CAD build for the part. Positions are in the model's coordinates, mm. A direction names the side the tool comes from. Coordinates: 2 decimals unless noted, no trailing zeros. Loops run counter-clockwise (first coordinate to the right, second up) from the corner with the lowest first, then second, coordinate; pieces in that order, holes last.
1) Which spindle directions (+Z, -Z, +X, -X, +Y, -Y) get a long thin tool onto all of the face, cutting with end or side? Do faces 1 (the flat face through (0, 0, 0)), 2 (the flat face through (-8.176, 3.933, -2.218)), 3 (the flat face through (0, 0, -4.5)). Say none if no direction does.
2) Pin check, flat tip, straight feed: pin 1 Ø12 at (x, y) = (-3.5, -5) entering from +Z. Stop position of the tip, or through.
3) Two-plate mould, pull along X, no slides. Class faces 4 (the flat face through (3.933, 8.176, -2.218)), 5 (the flat face through (-3.933, -8.176, -2.218)), 6 (the flat face through (-18, 0, -2)), 7 (the flat face through (-15, -17, 4)): +X half, -X half, draft (parallel to the pull), parting line (faces both ways), or undercut.
4) Saw through at B-B, the plane y = 11. Write the cut outline in (x, z).
5) Saw through at A-A, the plane z = -2. Give the number of separate pieces and of enclosed holes in the cut face, and give its area (3 significant figures).
6) Saw through at D-D, the plane y = -0.5. Write the cut outline in (x, z), and give its area (3 significant figures).
7) Wall check: line 1 along X through (y, z) = (-15, 2.4); line 2 along Y through (x, z) = (-15, -2.55). Give the ranges that are in metal, low to high.
8) Saw through at C-C, the plane x = -3. Write the cut outline in (y, z).
```python
from build123d import *
from build123d import SkipClean  # not in build123d's __all__

# Parameters (mm, degrees)
F1_W     = 36
F1_H     = 36
F2_DEPTH = 4.5
F3_DEPTH = 4


with BuildPart() as f2:
    # F1 (on Top) → F2 (new body)
    with BuildSketch(Plane.XY):
        Rectangle(F1_W, F1_H)
        with BuildLine():
            ThreePointArc((-15, 12.5), (-16.767766953, 16.767766953), (-12.5, 15))
            Line((-12.5, 15), (12.5, 15))
            ThreePointArc((12.5, 15), (15, 17.5), (17.5, 15))
            ThreePointArc((17.5, 15), (16.767766953, 13.232233047), (15, 12.5))
            Line((15, 12.5), (15, -12.5))
            ThreePointArc((15, -12.5), (16.767766953, -13.232233047), (17.5, -15))
            ThreePointArc((17.5, -15), (15, -17.5), (12.5, -15))
            Line((12.5, -15), (-12.5, -15))
            ThreePointArc((-12.5, -15), (-16.767766953, -16.767766953), (-15, -12.5))
            Line((-15, -12.5), (-15, 12.5))
        make_face(mode=Mode.SUBTRACT)
        with BuildLine():
            ThreePointArc((-13.232233047, 13.232233047), (-14.0432914191, 12.6903011687), (-15, 12.5))
            Line((-15, 12.5), (-15, -12.5))
            ThreePointArc((-15, -12.5), (-14.0432914191, -12.6903011687), (-13.232233047, -13.232233047))
            Line((-13.232233047, -13.232233047), (-12, -12))
            Line((-12, -12), (-12, -7.7573593129))
            Line((-12, -7.7573593129), (-12, 7.7573593129))
            Line((-12, 7.7573593129), (-12, 12))
            Line((-12, 12), (-13.232233047, 13.232233047))
        make_face()
        with BuildLine():
            Line((12.5, 15), (-12.5, 15))
            ThreePointArc((-12.5, 15), (-12.6903011687, 14.0432914191), (-13.232233047, 13.232233047))
            Line((-13.232233047, 13.232233047), (-12, 12))
            Line((-12, 12), (-7.7573593129, 12))
            Line((-7.7573593129, 12), (7.7573593129, 12))
            Line((7.7573593129, 12), (12, 12))
            Line((12, 12), (13.232233047, 13.232233047))
            ThreePointArc((13.232233047, 13.232233047), (12.6903011687, 14.0432914191), (12.5, 15))
        make_face()
        with BuildLine():
            Line((-12, -12), (-13.232233047, -13.232233047))
            ThreePointArc((-13.232233047, -13.232233047), (-12.6903011687, -14.0432914191), (-12.5, -15))
            Line((-12.5, -15), (12.5, -15))
            ThreePointArc((12.5, -15), (12.6903011687, -14.0432914191), (13.232233047, -13.232233047))
            Line((13.232233047, -13.232233047), (12, -12))
            Line((12, -12), (7.7573593129, -12))
            Line((7.7573593129, -12), (-7.7573593129, -12))
            Line((-7.7573593129, -12), (-12, -12))
        make_face()
        with BuildLine():
            ThreePointArc((15, 12.5), (14.0432914191, 12.6903011687), (13.232233047, 13.232233047))
            Line((13.232233047, 13.232233047), (12, 12))
            Line((12, 12), (12, 7.7573593129))
            Line((12, 7.7573593129), (12, -7.7573593129))
            Line((12, -7.7573593129), (12, -12))
            Line((12, -12), (13.232233047, -13.232233047))
            ThreePointArc((13.232233047, -13.232233047), (14.0432914191, -12.6903011687), (15, -12.5))
            Line((15, -12.5), (15, 12.5))
        make_face()
        Polygon((0, 0), (-12, 12), (-12, 7.7573593129), (-4.2426406871, 0), (-2.1213203436, -2.1213203436), align=None)
        Polygon((-7.7573593129, 12), (-12, 12), (0, 0), (2.1213203436, 2.1213203436), (0, 4.2426406871), align=None)
        Polygon((2.1213203436, 2.1213203436), (0, 0), (12, -12), (12, -7.7573593129), (4.2426406871, 0), align=None)
        Polygon((12, -12), (0, 0), (-2.1213203436, -2.1213203436), (0, -4.2426406871), (7.7573593129, -12), align=None)
        Polygon((-2.1213203436, -2.1213203436), (-12, -12), (-7.7573593129, -12), (0, -4.2426406871), align=None)
        Polygon((-12, -7.7573593129), (-12, -12), (-2.1213203436, -2.1213203436), (-4.2426406871, 0), align=None)
        Polygon((2.1213203436, 2.1213203436), (12, 12), (7.7573593129, 12), (0, 4.2426406871), align=None)
        Polygon((12, 7.7573593129), (12, 12), (2.1213203436, 2.1213203436), (4.2426406871, 0), align=None)
        with BuildLine():
            Line((-13.5, 15), (-12.5, 15))
            ThreePointArc((-12.5, 15), (-16.767766953, 16.767766953), (-15, 12.5))
            Line((-15, 12.5), (-15, 13.5))
            ThreePointArc((-15, 13.5), (-16.0606601718, 16.0606601718), (-13.5, 15))
        make_face()
        with BuildLine():
            ThreePointArc((17.5, 15), (15, 17.5), (12.5, 15))
            Line((12.5, 15), (13.5, 15))
            ThreePointArc((13.5, 15), (15, 16.5), (16.5, 15))
            ThreePointArc((16.5, 15), (16.0606601718, 13.9393398282), (15, 13.5))
            Line((15, 13.5), (15, 12.5))
            ThreePointArc((15, 12.5), (16.767766953, 13.232233047), (17.5, 15))
        make_face()
        with BuildLine():
            ThreePointArc((17.5, -15), (16.767766953, -13.232233047), (15, -12.5))
            Line((15, -12.5), (15, -13.5))
            ThreePointArc((15, -13.5), (16.0606601718, -13.9393398282), (16.5, -15))
            ThreePointArc((16.5, -15), (15, -16.5), (13.5, -15))
            Line((13.5, -15), (12.5, -15))
            ThreePointArc((12.5, -15), (15, -17.5), (17.5, -15))
        make_face()
        with BuildLine():
            Line((-15, -13.5), (-15, -12.5))
            ThreePointArc((-15, -12.5), (-16.767766953, -16.767766953), (-12.5, -15))
            Line((-12.5, -15), (-13.5, -15))
            ThreePointArc((-13.5, -15), (-16.0606601718, -16.0606601718), (-15, -13.5))
        make_face()
        with BuildLine():
            Line((-15, 13.5), (-15, 12.5))
            ThreePointArc((-15, 12.5), (-14.0432914191, 12.6903011687), (-13.232233047, 13.232233047))
            Line((-13.232233047, 13.232233047), (-13.9393398282, 13.9393398282))
            ThreePointArc((-13.9393398282, 13.9393398282), (-14.4259748515, 13.6141807012), (-15, 13.5))
        make_face()
        with BuildLine():
            ThreePointArc((-13.232233047, 13.232233047), (-12.6903011687, 14.0432914191), (-12.5, 15))
            Line((-12.5, 15), (-13.5, 15))
            ThreePointArc((-13.5, 15), (-13.6141807012, 14.4259748515), (-13.9393398282, 13.9393398282))
            Line((-13.9393398282, 13.9393398282), (-13.232233047, 13.232233047))
        make_face()
        with BuildLine():
            Line((13.9393398282, 13.9393398282), (13.232233047, 13.232233047))
            ThreePointArc((13.232233047, 13.232233047), (14.0432914191, 12.6903011687), (15, 12.5))
            Line((15, 12.5), (15, 13.5))
            ThreePointArc((15, 13.5), (14.4259748515, 13.6141807012), (13.9393398282, 13.9393398282))
        make_face()
        with BuildLine():
            Line((13.5, 15), (12.5, 15))
            ThreePointArc((12.5, 15), (12.6903011687, 14.0432914191), (13.232233047, 13.232233047))
            Line((13.232233047, 13.232233047), (13.9393398282, 13.9393398282))
            ThreePointArc((13.9393398282, 13.9393398282), (13.6141807012, 14.4259748515), (13.5, 15))
        make_face()
        with BuildLine():
            ThreePointArc((13.232233047, -13.232233047), (12.6903011687, -14.0432914191), (12.5, -15))
            Line((12.5, -15), (13.5, -15))
            ThreePointArc((13.5, -15), (13.6141807012, -14.4259748515), (13.9393398282, -13.9393398282))
            Line((13.9393398282, -13.9393398282), (13.232233047, -13.232233047))
        make_face()
        with BuildLine():
            Line((15, -13.5), (15, -12.5))
            ThreePointArc((15, -12.5), (14.0432914191, -12.6903011687), (13.232233047, -13.232233047))
            Line((13.232233047, -13.232233047), (13.9393398282, -13.9393398282))
            ThreePointArc((13.9393398282, -13.9393398282), (14.4259748515, -13.6141807012), (15, -13.5))
        make_face()
        with BuildLine():
            ThreePointArc((-12.5, -15), (-12.6903011687, -14.0432914191), (-13.232233047, -13.232233047))
            Line((-13.232233047, -13.232233047), (-13.9393398282, -13.9393398282))
            ThreePointArc((-13.9393398282, -13.9393398282), (-13.6141807012, -14.4259748515), (-13.5, -15))
            Line((-13.5, -15), (-12.5, -15))
        make_face()
        with BuildLine():
            ThreePointArc((-13.232233047, -13.232233047), (-14.0432914191, -12.6903011687), (-15, -12.5))
            Line((-15, -12.5), (-15, -13.5))
            ThreePointArc((-15, -13.5), (-14.4259748515, -13.6141807012), (-13.9393398282, -13.9393398282))
            Line((-13.9393398282, -13.9393398282), (-13.232233047, -13.232233047))
        make_face()
    extrude(amount=-F2_DEPTH)

    # F1 (on Top) → F3 (join)
    with BuildSketch(Plane.XY):
        with BuildLine():
            Line((-13.5, 15), (-12.5, 15))
            ThreePointArc((-12.5, 15), (-16.767766953, 16.767766953), (-15, 12.5))
            Line((-15, 12.5), (-15, 13.5))
            ThreePointArc((-15, 13.5), (-16.0606601718, 16.0606601718), (-13.5, 15))
        make_face()
        with BuildLine():
            Line((-15, 13.5), (-15, 12.5))
            ThreePointArc((-15, 12.5), (-14.0432914191, 12.6903011687), (-13.232233047, 13.232233047))
            Line((-13.232233047, 13.232233047), (-13.9393398282, 13.9393398282))
            ThreePointArc((-13.9393398282, 13.9393398282), (-14.4259748515, 13.6141807012), (-15, 13.5))
        make_face()
        with BuildLine():
            ThreePointArc((-13.232233047, 13.232233047), (-12.6903011687, 14.0432914191), (-12.5, 15))
            Line((-12.5, 15), (-13.5, 15))
            ThreePointArc((-13.5, 15), (-13.6141807012, 14.4259748515), (-13.9393398282, 13.9393398282))
            Line((-13.9393398282, 13.9393398282), (-13.232233047, 13.232233047))
        make_face()
        with BuildLine():
            ThreePointArc((17.5, 15), (15, 17.5), (12.5, 15))
            Line((12.5, 15), (13.5, 15))
            ThreePointArc((13.5, 15), (15, 16.5), (16.5, 15))
            ThreePointArc((16.5, 15), (16.0606601718, 13.9393398282), (15, 13.5))
            Line((15, 13.5), (15, 12.5))
            ThreePointArc((15, 12.5), (16.767766953, 13.232233047), (17.5, 15))
        make_face()
        with BuildLine():
            Line((13.9393398282, 13.9393398282), (13.232233047, 13.232233047))
            ThreePointArc((13.232233047, 13.232233047), (14.0432914191, 12.6903011687), (15, 12.5))
            Line((15, 12.5), (15, 13.5))
            ThreePointArc((15, 13.5), (14.4259748515, 13.6141807012), (13.9393398282, 13.9393398282))
        make_face()
        with BuildLine():
            Line((13.5, 15), (12.5, 15))
            ThreePointArc((12.5, 15), (12.6903011687, 14.0432914191), (13.232233047, 13.232233047))
            Line((13.232233047, 13.232233047), (13.9393398282, 13.9393398282))
            ThreePointArc((13.9393398282, 13.9393398282), (13.6141807012, 14.4259748515), (13.5, 15))
        make_face()
        with BuildLine():
            Line((-15, -13.5), (-15, -12.5))
            ThreePointArc((-15, -12.5), (-16.767766953, -16.767766953), (-12.5, -15))
            Line((-12.5, -15), (-13.5, -15))
            ThreePointArc((-13.5, -15), (-16.0606601718, -16.0606601718), (-15, -13.5))
        make_face()
        with BuildLine():
            ThreePointArc((-13.232233047, -13.232233047), (-14.0432914191, -12.6903011687), (-15, -12.5))
            Line((-15, -12.5), (-15, -13.5))
            ThreePointArc((-15, -13.5), (-14.4259748515, -13.6141807012), (-13.9393398282, -13.9393398282))
            Line((-13.9393398282, -13.9393398282), (-13.232233047, -13.232233047))
        make_face()
        with BuildLine():
            ThreePointArc((-12.5, -15), (-12.6903011687, -14.0432914191), (-13.232233047, -13.232233047))
            Line((-13.232233047, -13.232233047), (-13.9393398282, -13.9393398282))
            ThreePointArc((-13.9393398282, -13.9393398282), (-13.6141807012, -14.4259748515), (-13.5, -15))
            Line((-13.5, -15), (-12.5, -15))
        make_face()
        with BuildLine():
            Line((15, -13.5), (15, -12.5))
            ThreePointArc((15, -12.5), (14.0432914191, -12.6903011687), (13.232233047, -13.232233047))
            Line((13.232233047, -13.232233047), (13.9393398282, -13.9393398282))
            ThreePointArc((13.9393398282, -13.9393398282), (14.4259748515, -13.6141807012), (15, -13.5))
        make_face()
        with BuildLine():
            ThreePointArc((13.232233047, -13.232233047), (12.6903011687, -14.0432914191), (12.5, -15))
            Line((12.5, -15), (13.5, -15))
            ThreePointArc((13.5, -15), (13.6141807012, -14.4259748515), (13.9393398282, -13.9393398282))
            Line((13.9393398282, -13.9393398282), (13.232233047, -13.232233047))
        make_face()
        with BuildLine():
            ThreePointArc((17.5, -15), (16.767766953, -13.232233047), (15, -12.5))
            Line((15, -12.5), (15, -13.5))
            ThreePointArc((15, -13.5), (16.0606601718, -13.9393398282), (16.5, -15))
            ThreePointArc((16.5, -15), (15, -16.5), (13.5, -15))
            Line((13.5, -15), (12.5, -15))
            ThreePointArc((12.5, -15), (15, -17.5), (17.5, -15))
        make_face()
    with SkipClean():  # cleaning this boolean's faces spoils the solid; the shape is the same uncleaned
        extrude(amount=F3_DEPTH)


solid = f2.part
```
Data:
1. face 1: +Z
1. face 2: +Z, -Z
1. face 3: -Z, +X, -X, +Y, -Y
2. pin 1: stops at z = 0
3. face 4: undercut
3. face 5: undercut
3. face 6: -X half
3. face 7: draft
4. outline: (-18, -4.5) - (-6.76, -4.5) - (-6.76, 0) - (-18, 0) - close; (6.76, -4.5) - (18, -4.5) - (18, 0) - (6.76, 0) - close
5. separate pieces: 1
5. enclosed holes: 8
5. area: 1,030 mm2
6. outline: (-18, -4.5) - (-12, -4.5) - (-12, 0) - (-18, 0) - close; (-4.74, -4.5) - (4.74, -4.5) - (4.74, 0) - (-4.74, 0) - close; (12, -4.5) - (18, -4.5) - (18, 0) - (12, 0) - close
6. area: 96.7 mm2
7. line 1: x = -17.5 to -16.5, -13.5 to -12.5, 12.5 to 13.5, 16.5 to 17.5
7. line 2: y = -18 to -16.5, -13.5 to 13.5, 16.5 to 18
8. outline: (-18, -4.5) - (-12, -4.5) - (-12, 0) - (-18, 0) - close; (-7.24, -4.5) - (7.24, -4.5) - (7.24, 0) - (-7.24, 0) - close; (12, -4.5) - (18, -4.5) - (18, 0) - (12, 0) - close
